```python
from build123d import *

# Parameters (mm, degrees)
CROQUIS1_W              = 10
CROQUIS1_H              = 8
CROQUIS1_R              = 1.5
SALIENTE_EXTRUIR1_DEPTH = 4
CROQUIS2_R              = 2.85
CORTAR_EXTRUIR1_DEPTH   = 1.65


with BuildPart() as part:
    # Croquis1 → Saliente-Extruir1 (new body)
    # profile 1 of 2: a face of its own
    with BuildSketch(Plane.XY):
        with Locations((-39.5, 69)):
            Rectangle(CROQUIS1_W, CROQUIS1_H)
        with Locations((-39.5, 69)):
            Circle(CROQUIS1_R, mode=Mode.SUBTRACT)
    # profile 2 of 2: a face of its own
    with BuildSketch(Plane.XY):
        with Locations((-49.5, 69)):
            Rectangle(CROQUIS1_W, CROQUIS1_H)
        with Locations((-49.5, 69)):
            Circle(CROQUIS1_R, mode=Mode.SUBTRACT)
    extrude(amount=SALIENTE_EXTRUIR1_DEPTH)

    # Croquis2 → Cortar-Extruir1 (cut)
    with BuildSketch(Plane.XY.offset(4)):
        with Locations((-49.5, 69)):
            Circle(CROQUIS2_R)
        with Locations((-39.5, 69)):
            Circle(CROQUIS2_R)
    extrude(amount=-CORTAR_EXTRUIR1_DEPTH, mode=Mode.SUBTRACT)


solid = part.part
```
Source: CAD feature listing. Evaluate the final solid. Frame: model axes, mm. A direction names the side the tool comes from. Give positions to 0.01 mm unless a question says otherwise; leave off trailing zeros. Loops run counter-clockwise (first coordinate to the right, second up) from the corner with the lowest first, then second, coordinate; pieces in that order, holes last. Notation, with made-up numbers: (-24, -14.75) -> (-12, -14.75) arc R21 ccw to (-12, -2.75) -> close; hole circle Ø5 at (22.5, -1). An arc over 180 degrees is marked (long way). Use a Markdown table: item, result. Add a question column.
(1) Section query D-D (y = 70.25). Output: boundary loops of the cut face in (x, z).
(2) Ray query, line 1 (X direction, y = 69, z = 1.85); line 2 (Y direction, x = -49.5, z = 3.3); line 3 (Y direction, x = -49.5, z = 1.25). Return the intervals inside material, ascending.
(3) Access query for faces 5 (the face through (-49.871, 71.826, 3.187)), 6 (the face through (-45, 65, 2)). Directions: +Z, -Z, +X, -X, +Y, -Y. A direction counts if a zero-diameter tool reaches every point of the face in a straight line with its end or side. Return the directions, or none.
(4) Section query C-C (z = 3.45). Output: boundary loops of the cut face in (x, y).
(5) Pull-direction query (Y, two-part tool) for faces 1 (the face through (-45, 73, 2)), 2 (the face through (-41, 69, 1)), 3 (the face through (-45, 69, 4)), 4 (the face through (-38, 68, 2.35)); classes: +Y half, -Y half, draft (parallel to the pull), parting line (faces both ways), or undercut.
(6) Section query A-A (x = -39.5). Output: boundary loops of the cut face in (y, z).
(7) First-contact query: pin 1 Ø3 at (x, y) = (-49.5, 70) entering from +Z. Flat tip, straight axial feed; report the tip coordinate or a pass-through.
(8) Section query B-B (y = 69). Output: boundary loops of the cut face in (x, z).
Checked values:
| question | item | result |
|---|---|---|
| 1 | outline | (-54.5, 0) -> (-50.33, 0) -> (-50.33, 2.35) -> (-52.06, 2.35) -> (-52.06, 4) -> (-54.5, 4) -> close; (-48.67, 0) -> (-40.33, 0) -> (-40.33, 2.35) -> (-42.06, 2.35) -> (-42.06, 4) -> (-46.94, 4) -> (-46.94, 2.35) -> (-48.67, 2.35) -> close; (-38.67, 0) -> (-34.5, 0) -> (-34.5, 4) -> (-36.94, 4) -> (-36.94, 2.35) -> (-38.67, 2.35) -> close |
| 2 | line 1 | -54.5 to -51, -48 to -41, -38 to -34.5 |
| 2 | line 2 | 65 to 66.15, 71.85 to 73 |
| 2 | line 3 | 65 to 67.5, 70.5 to 73 |
| 3 | face 5 | +Z |
| 3 | face 6 | +Z, -Z, +X, -X, -Y |
| 4 | outline | (-54.5, 65) -> (-34.5, 65) -> (-34.5, 73) -> (-54.5, 73) -> close; hole circle Ø5.7 at (-49.5, 69); hole circle Ø5.7 at (-39.5, 69) |
| 5 | face 1 | +Y half |
| 5 | face 2 | undercut |
| 5 | face 3 | draft |
| 5 | face 4 | undercut |
| 6 | outline | (65, 0) -> (67.5, 0) -> (67.5, 2.35) -> (66.15, 2.35) -> (66.15, 4) -> (65, 4) -> close; (70.5, 0) -> (73, 0) -> (73, 4) -> (71.85, 4) -> (71.85, 2.35) -> (70.5, 2.35) -> close |
| 7 | pin 1 | z = 2.35 |
| 8 | outline | (-54.5, 0) -> (-51, 0) -> (-51, 2.35) -> (-52.35, 2.35) -> (-52.35, 4) -> (-54.5, 4) -> close; (-48, 0) -> (-41, 0) -> (-41, 2.35) -> (-42.35, 2.35) -> (-42.35, 4) -> (-46.65, 4) -> (-46.65, 2.35) -> (-48, 2.35) -> close; (-38, 0) -> (-34.5, 0) -> (-34.5, 4) -> (-36.65, 4) -> (-36.65, 2.35) -> (-38, 2.35) -> close |
